from build123d import *

# Parameters (mm, degrees)
F0_R          = 49.75
F0_R_2        = 48.25
F1_DEPTH      = 73
F3_R          = 2.5
F4_DEPTH      = 49.751
F4_DEPTH_BACK = 49.751
F2_R          = 2.5
F5_DEPTH      = 49.7510001
F5_DEPTH_BACK = 49.7510001


with BuildPart() as f1:
    # F0 (on Front) → F1 (new body, symmetric)
    with BuildSketch(Plane.XZ):
        Circle(F0_R)
        Circle(F0_R_2, mode=Mode.SUBTRACT)
    extrude(amount=F1_DEPTH, both=True)

    # F3 (on Right) → F4 (cut, two sides)
    with BuildSketch(Plane.YZ) as f4_sk:
        with Locations((63, 0)):
            Circle(F3_R)
    extrude(amount=F4_DEPTH, mode=Mode.SUBTRACT)
    extrude(f4_sk.sketch, amount=-F4_DEPTH_BACK, mode=Mode.SUBTRACT)

    # F2 (on Top) → F5 (cut, two sides)
    with BuildSketch(Plane.XY) as f5_sk:
        with Locations((0, 63)):
            Circle(F2_R)
    extrude(amount=-F5_DEPTH, mode=Mode.SUBTRACT)
    extrude(f5_sk.sketch, amount=F5_DEPTH_BACK, mode=Mode.SUBTRACT)


solid = f1.part
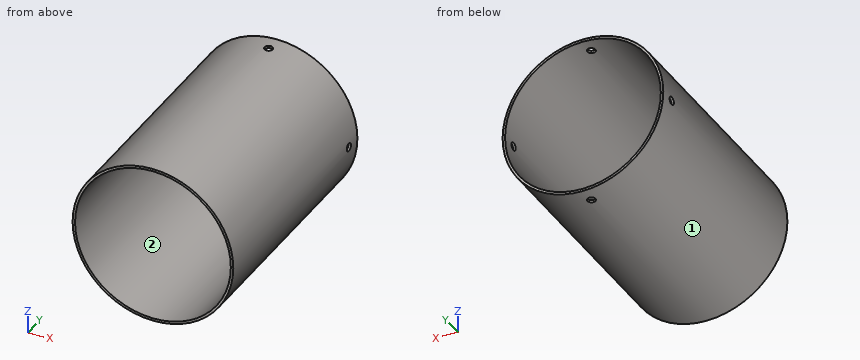
CAD build for the part. Positions are in the model's coordinates, mm. Face numbers are marked on the shaded views. Round coordinates to 2 decimals unless told otherwise and drop trailing zeros. Loops run counter-clockwise (first coordinate to the right, second up) from the corner with the lowest first, then second, coordinate; pieces in that order, holes last. Notation, with made-up numbers: (83, 3) - (96, 3) arc R15 ccw to (96, 16) - close; hole circle Ø4 at (80.5, 4.5). An arc over 180 degrees is marked (long way). Put each result on its own line as item: value.
1. Wall check: line 1 (Y direction, x = 0, z = -48.8); line 2 (X direction, y = -41, z = 25); line 3 (Z direction, x = 10, y = -39). Give the ranges that are in metal, low to high.
Geometry check:
line 1: -73 to 60.5, 65.5 to 73
line 2: -43.01 to -41.27, 41.27 to 43.01
line 3: -48.73 to -47.2, 47.2 to 48.73
2. Slice it at A-A on z = 0. List the corners of the cut face in (x, y), and give its area (3 significant figures).
Geometry check:
outline: (-49.75, -73) - (-48.25, -73) - (-48.25, 60.5) - (-49.75, 60.5) - close; (-49.75, 65.5) - (-48.25, 65.5) - (-48.25, 73) - (-49.75, 73) - close; (48.25, -73) - (49.75, -73) - (49.75, 60.5) - (48.25, 60.5) - close; (48.25, 65.5) - (49.75, 65.5) - (49.75, 73) - (48.25, 73) - close
area: 423 mm²
3. Pin check, flat tips, straight feed: P1, Ø8, axis at y = -6.5, z = 7.5, coming from the -X side; P2, Ø12, axis at x = -22, y = 27, coming from the +Z side; P3, Ø5, axis at x = 38.5, y = -49, coming from the +Z side. Stop position of each tip, or through.
Geometry check:
P1: x = -49.63
P2: z = 47.11
P3: z = 34.34
4. Slice it at D-D on y = -27.5. List the corners of the cut face in (x, z), and give its area (3 significant figures).
Geometry check:
outline: circle Ø99.5 at (0, 0); hole circle Ø96.5 at (0, 0)
area: 462 mm²
5. Slice it at C-C on z = -30.5. List the corners of the cut face in (x, y).
Geometry check:
outline: (-39.3, -73) - (-37.39, -73) - (-37.39, 73) - (-39.3, 73) - close; (37.39, -73) - (39.3, -73) - (39.3, 73) - (37.39, 73) - close
6. Two-plate mould, pull along X, no slides. Class the marked faces 1 and 2: released by +X, released by -X, zero draft, split by the parting line, or undercut.
Geometry check:
face 1: split by the parting line
face 2: undercut
7. Slice it at B-B on x = 0. List the corners of the cut face in (y, z).
Geometry check:
outline: (-73, -49.75) - (60.5, -49.75) - (60.5, -48.25) - (-73, -48.25) - close; (-73, 48.25) - (60.5, 48.25) - (60.5, 49.75) - (-73, 49.75) - close; (65.5, -49.75) - (73, -49.75) - (73, -48.25) - (65.5, -48.25) - close; (65.5, 48.25) - (73, 48.25) - (73, 49.75) - (65.5, 49.75) - close
